from build123d import *

# Parameters (mm, degrees)
SKETCH3_R           = 2
BOSS_EXTRUDE1_DEPTH = 4
FILLET1_R           = 10
SKETCH4_R           = 4
SKETCH4_R_2         = 2
BOSS_EXTRUDE2_DEPTH = 3


with BuildPart() as part:
    # Sketch3 → Boss-Extrude1 (new body)
    with BuildSketch(Plane.XY):
        Polygon((-42.75, 8.482081222), (-42.75, -16), (-34.5, -16), (-34.5, -57.1), (-42.75, -57.1), (-42.75, -92.85), (42.75, -92.85), (42.75, -57.1), (34.5, -57.1), (34.5, -16), (42.75, -16), (42.75, 8.482081222), (0, 27.552713192), align=None)
        with Locations((-38.25, 5)):
            Circle(SKETCH3_R, mode=Mode.SUBTRACT)
        with Locations((-38.25, -87.85)):
            Circle(SKETCH3_R, mode=Mode.SUBTRACT)
        with Locations(Location((38.25, -87.85, 0), (0, 0, 180))):
            Circle(SKETCH3_R, mode=Mode.SUBTRACT)
        with Locations(Location((38.25, 5, 0), (0, 0, 180))):
            Circle(SKETCH3_R, mode=Mode.SUBTRACT)
    extrude(amount=BOSS_EXTRUDE1_DEPTH)

    # Fillet1
    # the kernel refuses this fillet: 10 mm, written as the material it adds along each edge
    with BuildSketch(Plane(origin=(34.5, -57.1, 0), x_dir=(1, 0, 0), z_dir=(0, 0, 1)), Plane(origin=(-34.5, -16, 0), x_dir=(-1, 0, 0), z_dir=(0, 0, 1))) as fillet1_piece_1:
        with BuildLine():
            CenterArc((10, 9.845684334), FILLET1_R, 180, 79.921341892)
            Line((0, 9.845684334), (-0.2, 9.845684334))
            Line((-0.2, 9.845684334), (-0.2, 0))
            Line((-0.2, 0), (0, -0.2))
            ThreePointArc((0, -0.2), (4.125, -0.2), (8.215, -0.196913687))
            Line((8.215, -0.196913687), (8.25, 0))
        make_face()
    extrude(amount=4)
    with BuildSketch(Plane(origin=(34.5, -16, 0), x_dir=(0, -1, 0), z_dir=(0, 0, 1)), Plane(origin=(-34.5, -57.1, 0), x_dir=(0, 1, 0), z_dir=(0, 0, 1))) as fillet1_piece_2:
        with BuildLine():
            CenterArc((9.845684334, 10), FILLET1_R, 190.078658108, 79.921341892)
            Line((0, 8.25), (-0.196913687, 8.215))
            ThreePointArc((-0.196913687, 8.215), (-0.2, 4.125), (-0.2, 0))
            Line((-0.2, 0), (0, -0.2))
            Line((0, -0.2), (9.845684334, -0.2))
            Line((9.845684334, -0.2), (9.845684334, 0))
        make_face()
    extrude(amount=4)

    # Sketch4 → Boss-Extrude2 (add)
    # profile 1 of 2: a face of its own
    with BuildSketch(Plane.XY.offset(4)):
        with Locations(Location((38.25, -87.85, 0), (0, 0, 180))):
            Circle(SKETCH4_R)
        with Locations(Location((38.25, -87.85, 0), (0, 0, 180))):
            Circle(SKETCH4_R_2, mode=Mode.SUBTRACT)
    # profile 2 of 2: a face of its own
    with BuildSketch(Plane.XY.offset(4)):
        with Locations(Location((-38.25, -87.85, 0), (0, 0, 180))):
            Circle(SKETCH4_R)
        with Locations((-38.25, -87.85)):
            Circle(SKETCH4_R_2, mode=Mode.SUBTRACT)
    extrude(amount=BOSS_EXTRUDE2_DEPTH)


solid = part.part
Could you check a few things on this model? Use its own coordinates, in mm. A direction names the side the tool comes from. Give positions to 0.01 mm unless a question says otherwise; leave off trailing zeros. Order: outer loops, then holes, each group sorted by start corner. A loop starts at its lowest first (then second) coordinate and runs counter-clockwise, first axis right, second up.
1. Suppose I cut it at C-C (x = -38.25). Write out the boundary of the cut face in (y, z).
Answers below:
outline: (-92.85, 0) - (-89.85, 0) - (-89.85, 7) - (-91.85, 7) - (-91.85, 4) - (-92.85, 4) - close; (-85.85, 0) - (-55.06, 0) - (-55.06, 4) - (-83.85, 4) - (-83.85, 7) - (-85.85, 7) - close; (-18.04, 0) - (3, 0) - (3, 4) - (-18.04, 4) - close; (7, 0) - (10.49, 0) - (10.49, 4) - (7, 4) - close
2. For pin 1 (12 mm diameter, centred on x = 23, y = -28.5, fed in from +Z); pin 2 (2.5 mm diameter, centred on x = 38.25, y = 5, fed in from +Z); pin 3 (3 mm diameter, centred on x = 2.5, y = -20, fed in from -Z); pin 4 (4 mm diameter, centred on y = -23.5, z = 5, fed in from -X), each with a flat end and sliding along its axis, tell me the tip position at first contact or that it passes through.
Answers below:
pin 1: stops at z = 4
pin 2: passes through
pin 3: stops at z = 0
pin 4: stops at x = -35.37
3. I need wall thicknesses on L1, parallel to Y at x = 38.25, z = 2.85; L2, parallel to Y at x = 38, z = 1.5; L3, parallel to Y at x = 38.25, z = 5.25. Which ranges of each line are inside material? Lowest first, please.
Answers below:
L1: y = -92.85 to -89.85, -85.85 to -55.06, -18.04 to 3, 7 to 10.49
L2: y = -92.85 to -89.83, -85.87 to -54.85, -18.25 to 3.02, 6.98 to 10.6
L3: y = -91.85 to -89.85, -85.85 to -83.85
4. Thinking about a two-plate mould opening in X: for faces 1 (the cylindrical face through (-37.729, -91.816, 5.479)), 2 (the flat face through (-34.5, -36, 2)), 3 (the flat face through (34.5, -37, 2)), which applies, +X half, -X half, draft (parallel to the pull), parting line (faces both ways), or undercut?
Answers below:
face 1: undercut
face 2: -X half
face 3: +X half
5. Which directions (+Z, -Z, +X, -X, +Y, -Y) give clear straight access to the entire face, cutting with the end or side of a thin tool? Please do faces 4 (the cylindrical face through (-36.77, -19.5, 1.97)), 5 (the cylindrical face through (36.898, -19.349, 1.972)), 6 (the cylindrical face through (38.771, -91.816, 5.479)), 7 (the flat face through (-42.75, -4, 2)), 8 (the flat face through (42.75, -75, 2)).
Answers below:
face 4: +Z, -Z, -X
face 5: +Z, -Z, +X
face 6: +Z
face 7: +Z, -Z, -X, +Y, -Y
face 8: +Z, -Z, +X, +Y, -Y
6. Suppose I cut it at D-D (y = -45.5). Write out the boundary of the cut face in (x, z), plus the area to 3 significant figures.
Answers below:
outline: (-34.5, 0) - (34.5, 0) - (34.5, 4) - (-34.5, 4) - close
area: 276 mm2
7. Suppose I cut it at A-A (y = 5). Write out the boundary of the cut face in (x, z), plus the area to 3 significant figures.
Answers below:
outline: (-42.75, 0) - (-40.25, 0) - (-40.25, 4) - (-42.75, 4) - close; (-36.25, 0) - (36.25, 0) - (36.25, 4) - (-36.25, 4) - close; (40.25, 0) - (42.75, 0) - (42.75, 4) - (40.25, 4) - close
area: 310 mm2
8. Suppose I cut it at B-B (z = 5.5). Write out the boundary of the cut face in (x, y), plus the area to 3 significant figures.
Answers below:
outline: circle Ø8 at (-38.25, -87.85); circle Ø8 at (38.25, -87.85); hole circle Ø4 at (-38.25, -87.85); hole circle Ø4 at (38.25, -87.85)
area: 75.4 mm2
